Part model, mm, in its own coordinate system. Coordinates: 2 decimals unless noted, no trailing zeros. Write each loop counter-clockwise with the first axis right and the second up, starting at its lowest first coordinate (ties: lowest second). Pieces come first, ordered by that corner, then holes. Notation, with made-up numbers: (-31.75, 66) -> (4.25, 66) arc R29 ccw to (4.25, 96) -> close; hole circle Ø9 at (72, -13). An arc over 180 degrees is marked (long way). Write item = value, one per line. Start each with the question number.
Q1. Pull direction Z, two halves, no side cores. Call faces 1 (the flat face through (6.35, 63, 1)), 2 (the cylindrical face through (1.907, 31.306, 6.057)), 3 (the cylindrical face through (-5.94, 10.76, 1.35)): released by +Z, released by -Z, zero draft, split by the parting line, or undercut.
Q2. Pin check, flat tips, straight feed: P1, Ø1, axis at x = 4, y = 45, coming from the -Z side; P2, Ø5, axis at y = 35.5, z = 3, coming from the -X side; P3, Ø1, axis at x = -3, y = 27, coming from the +Z side. Stop position of each tip, or through.
Q3. Band-saw the part on B-B, the plane z = 3.75. List the corners of the cut face in (x, y).
Q4. Band-saw the part on C-C, the plane y = 19.5. List the corners of the cut face in (x, z).
Q5. Band-saw the part on A-A, the plane x = 0. List the corners of the cut face in (y, z), plus the area to 3 significant figures.
Q6. Probe line 1 (Y direction, x = -6, z = 0); line 2 (X direction, y = 14.5, z = 0); line 3 (X direction, y = 28, z = -4.5). List the from-to ranges inside material, lowest first.
from build123d import *
from build123d.topology import SkipClean

# Parameters (mm, degrees)
SKETCH1_R                = 6.35
SKETCH1_R_2              = 5.842
BOSS_EXTRUDE1_DEPTH      = 63.5
SKETCH2_R                = 0.8001
CUT_EXTRUDE1_DEPTH       = 66.068137364
BOSS_EXTRUDE2_REACH      = 67.068
BOSS_EXTRUDE2_END_RADIUS = 6.35
SKETCH3_W                = 2.6162
SKETCH3_H                = 2.6162
SKETCH3_R                = 0.8001
SKETCH4_R                = 1.8288
CUT_EXTRUDE2_DEPTH       = 66.068137491
BOSS_EXTRUDE3_REACH      = 67.068
BOSS_EXTRUDE3_END_RADIUS = 6.35
SKETCH5_W                = 5.08
SKETCH5_H                = 5.08
SKETCH5_R                = 1.8288


with BuildPart() as part:
    # Sketch1 → Boss-Extrude1 (new body)
    with BuildSketch(Plane(origin=(0, 0, 0), x_dir=(1, 0, 0), z_dir=(0, 1, 0))):
        with Locations(Location((0, 0, 0), (0, 0, 270))):
            Circle(SKETCH1_R)
        with Locations(Location((0, 0, 0), (0, 0, 270))):
            Circle(SKETCH1_R_2, mode=Mode.SUBTRACT)
    extrude(amount=BOSS_EXTRUDE1_DEPTH)

    # Sketch2 → Cut-Extrude1 (cut, through all)
    with BuildSketch(Plane(origin=(6.35, 0, 0), x_dir=(0, 0, -1), z_dir=(1, 0, 0))):
        with Locations((0, 62.1919)):
            Circle(SKETCH2_R)
    extrude(amount=-CUT_EXTRUDE1_DEPTH, mode=Mode.SUBTRACT)

    # Boss-Extrude2: up to this cylinder (the profile starts outside it)
    with SkipClean():  # the faces are left unmerged after this step: merging them gives an invalid solid
        boss_extrude2_end = Plane(origin=(0, 60.920799, 0), z_dir=(0, -1, 0)) * Cylinder(BOSS_EXTRUDE2_END_RADIUS, 147.836, mode=Mode.PRIVATE)
        # Sketch3 → Boss-Extrude2 (add, up to the surface)
        with BuildSketch(Plane(origin=(6.35, 0, 0), x_dir=(0, 0, -1), z_dir=(1, 0, 0)), mode=Mode.PRIVATE) as boss_extrude2_sk1:
            with Locations((0, 62.1919)):
                Rectangle(SKETCH3_W, SKETCH3_H)
            with Locations((0, 62.1919)):
                Circle(SKETCH3_R, mode=Mode.SUBTRACT)
        boss_extrude2_tool1 = extrude(boss_extrude2_sk1.sketch, amount=-BOSS_EXTRUDE2_REACH, mode=Mode.PRIVATE) - boss_extrude2_end
        add(boss_extrude2_tool1.solids().sort_by_distance((6.35, 60.920799, 0))[0])
        add(boss_extrude2_tool1.solids().sort_by_distance((6.35, 60.920799, 0))[1])

    # Sketch4 → Cut-Extrude2 (cut, through all)
    with BuildSketch(Plane(origin=(6.35, 0, 0), x_dir=(0, 0, -1), z_dir=(1, 0, 0))):
        with Locations((0, 9.525)):
            Circle(SKETCH4_R)
    extrude(amount=-CUT_EXTRUDE2_DEPTH, mode=Mode.SUBTRACT)

    # Boss-Extrude3: up to this cylinder (the profile starts outside it)
    with SkipClean():  # the faces are left unmerged after this step: merging them gives an invalid solid
        boss_extrude3_end = Plane(origin=(0, 7.056842, 0), z_dir=(0, -1, 0)) * Cylinder(BOSS_EXTRUDE3_END_RADIUS, 147.836, mode=Mode.PRIVATE)
        # Sketch5 → Boss-Extrude3 (add, up to the surface)
        with BuildSketch(Plane(origin=(6.35, 0, 0), x_dir=(0, 0, -1), z_dir=(1, 0, 0)), mode=Mode.PRIVATE) as boss_extrude3_sk1:
            with Locations((0, 9.525)):
                Rectangle(SKETCH5_W, SKETCH5_H)
            with Locations((0, 9.525)):
                Circle(SKETCH5_R, mode=Mode.SUBTRACT)
        boss_extrude3_tool1 = extrude(boss_extrude3_sk1.sketch, amount=-BOSS_EXTRUDE3_REACH, mode=Mode.PRIVATE) - boss_extrude3_end
        add(boss_extrude3_tool1.solids().sort_by_distance((6.35, 7.056842, 0))[0])
        add(boss_extrude3_tool1.solids().sort_by_distance((6.35, 7.056842, 0))[1])


solid = part.part
Ans:
q1.face_1 = zero draft
q1.face_2 = split by the parting line
q1.face_3 = undercut
q2.P1 = -5.3
q2.P2 = -6.33
q2.P3 = 5.84
q3.outline = (-5.12, 0) -> (-4.48, 0) -> (-4.48, 63.5) -> (-5.12, 63.5) -> close; (4.48, 0) -> (5.12, 0) -> (5.12, 63.5) -> (4.48, 63.5) -> close
q4.outline = circle Ø12.7 at (0, 0); hole circle Ø11.68 at (0, 0)
q5.outline = (0, -6.35) -> (63.5, -6.35) -> (63.5, -5.84) -> (0, -5.84) -> close; (0, 5.84) -> (63.5, 5.84) -> (63.5, 6.35) -> (0, 6.35) -> close
q5.area = 64.5 mm2
q6.line_1 = 0 to 7.7, 11.35 to 61.39, 62.99 to 63.5
q6.line_2 = -6.35 to -5.84, 5.84 to 6.35
q6.line_3 = -4.48 to -3.73, 3.73 to 4.48
